Part model, mm, in its own coordinate system. A direction names the side the tool comes from. Give positions to 0.01 mm unless a question says otherwise; leave off trailing zeros. Loops run counter-clockwise (first coordinate to the right, second up) from the corner with the lowest first, then second, coordinate; pieces in that order, holes last. Notation, with made-up numbers: M -29.75,-3 L -5.75,-3 A15 ccw -5.75,26 Z; hole C -37,59.25 d2. An arc over 180 degrees is marked long. Answer in a Markdown table with one row per item.
from build123d import *

# Parameters (mm, degrees)
EXTRUDE_1_DEPTH     = 3.2
SKETCH_2_R          = 12.5
SKETCH_2_R_2        = 1.6
SKETCH_2_R_3        = 1.5
SKETCH_2_R_4        = 6.45
CUT_EXTRUDE_1_DEPTH = 3.2
FILLET_1_R          = 2
FILLET_2_R          = 1


# Read off the part's stored shape, not the designer's step: 凸台-拉伸1
with BuildPart() as part:
    # 凸台-拉伸1 outline → 凸台-拉伸1 (new body)
    with BuildSketch(Plane(origin=(0, 0, 0), x_dir=(1, 0, 0), z_dir=(0, 1, 0))):
        Polygon((-55, -0.171572875), (-66.828427125, -12), (-73, -12), (-73, -30), (73, -30), (73, -12), (66.828427125, -12), (55, -0.171572875), (55, 30), (-55, 30), align=None)
        Polygon((-64, -12), (-55, -3), (-55, -12), align=None, mode=Mode.SUBTRACT)
        Polygon((55, -12), (55, -3), (64, -12), align=None, mode=Mode.SUBTRACT)
    extrude(amount=EXTRUDE_1_DEPTH)

    # 草图2 → 切除-拉伸1 (cut)
    with BuildSketch(Plane(origin=(0, 3.2, 0), x_dir=(1, 0, 0), z_dir=(0, 1, 0))):
        with Locations(Location((0, -9.443650814, 0), (0, 0, 270))):
            Circle(SKETCH_2_R)
        with Locations(Location((15.556349186, -25, 0), (0, 0, 270))):
            Circle(SKETCH_2_R_2)
        with Locations(Location((15.556349186, 6.112698372, 0), (0, 0, 270))):
            Circle(SKETCH_2_R_2)
        with Locations(Location((-15.556349186, 6.112698372, 0), (0, 0, 270))):
            Circle(SKETCH_2_R_2)
        with Locations(Location((-15.556349186, -25, 0), (0, 0, 270))):
            Circle(SKETCH_2_R_2)
        with Locations(Location((-52.5, 20, 0), (0, 0, 270))):
            Circle(SKETCH_2_R_3)
        with Locations(Location((-52.5, -20, 0), (0, 0, 270))):
            Circle(SKETCH_2_R_3)
        with Locations(Location((52.5, -20, 0), (0, 0, 270))):
            Circle(SKETCH_2_R_3)
        with Locations(Location((52.5, 20, 0), (0, 0, 270))):
            Circle(SKETCH_2_R_3)
        with Locations(Location((-64, -21, 0), (0, 0, 270))):
            Circle(SKETCH_2_R_4)
        with Locations(Location((64, -21, 0), (0, 0, 270))):
            Circle(SKETCH_2_R_4)
        with Locations(Location((42, 20, 0), (0, 0, 270))):
            Circle(SKETCH_2_R_3)
        with Locations(Location((42, 12, 0), (0, 0, 270))):
            Circle(SKETCH_2_R_3)
        with Locations(Location((-42, 12, 0), (0, 0, 270))):
            Circle(SKETCH_2_R_3)
        with Locations(Location((-42, 20, 0), (0, 0, 270))):
            Circle(SKETCH_2_R_3)
        with Locations(Location((42, -11, 0), (0, 0, 270))):
            Circle(SKETCH_2_R_3)
        with Locations(Location((-42, -11, 0), (0, 0, 270))):
            Circle(SKETCH_2_R_3)
        with Locations(Location((-28.065, 27, 0), (0, 0, 270))):
            Circle(SKETCH_2_R_3)
        with Locations(Location((28.065, 27, 0), (0, 0, 270))):
            Circle(SKETCH_2_R_3)
        with Locations(Location((-28.065, -16.18, 0), (0, 0, 270))):
            Circle(SKETCH_2_R_3)
        with Locations(Location((28.065, -16.18, 0), (0, 0, 270))):
            Circle(SKETCH_2_R_3)
        with Locations(Location((-28.769, -27.5, 0), (0, 0, 270))):
            Circle(SKETCH_2_R_3)
        with Locations(Location((28.769, -27.5, 0), (0, 0, 270))):
            Circle(SKETCH_2_R_3)
        with Locations(Location((-44.769, -20, 0), (0, 0, 270))):
            Circle(SKETCH_2_R_3)
        with Locations(Location((44.769, -20, 0), (0, 0, 270))):
            Circle(SKETCH_2_R_3)
    extrude(amount=-CUT_EXTRUDE_1_DEPTH, mode=Mode.SUBTRACT)

    # 圆角1
    fillet_1_edges = [part.edges().sort_by_distance(p)[0] for p in [
        (-66.828427125, 1.6, 12),
        (-55, 1.6, 0.171572875),
        (-55, 1.6, -30),
        (55, 1.6, -30),
        (55, 1.6, 0.171572875),
        (66.828427125, 1.6, 12),
        (73, 1.6, 12),
        (73, 1.6, 30),
        (-73, 1.6, 30),
        (-73, 1.6, 12),
    ]]
    fillet(fillet_1_edges, radius=FILLET_1_R)

    # 圆角2
    fillet_2_edges = [part.edges().sort_by_distance(p)[0] for p in [
        (-64, 1.6, 12),
        (-55, 1.6, 12),
        (-55, 1.6, 3),
        (55, 1.6, 3),
        (55, 1.6, 12),
        (64, 1.6, 12),
    ]]
    fillet(fillet_2_edges, radius=FILLET_2_R)


solid = part.part
(1) Pin check, flat tips, straight feed: pin 1 Ø7.5 at (x, z) = (-64, 21) entering from -Y; pin 2 Ø1.6 at (y, z) = (2, -15.5) entering from +X. Stop position of each tip, or through.
Recorded:
| item | result |
|---|---|
| pin 1 | passes through |
| pin 2 | stops at x = 55 |
(2) Saw through at C-C (x = -64). Write the cut outline in (y, z), plus the area to 3 significant figures.
Recorded:
| item | result |
|---|---|
| outline | M 0,9.17 L 3.2,9.17 L 3.2,14.55 L 0,14.55 Z; M 0,27.45 L 3.2,27.45 L 3.2,30 L 0,30 Z |
| area | 25.4 mm^2 |
(3) Pull direction Z, two halves, no side cores. Call faces 3 (the face through (55, 2, 8)), 4 (the face through (-1, 0, -7)), 5 (the face through (-1, 2, 30)): +Z half, -Z half, draft (parallel to the pull), parting line (faces both ways), or undercut.
Recorded:
| item | result |
|---|---|
| face 3 | undercut |
| face 4 | draft |
| face 5 | +Z half |
(4) Which spindle directions (+Z, -Z, +X, -X, +Y, -Y) get a long thin tool onto all of the face, cutting with end or side? Do faces 1 (the face through (73, 2, 21)), 2 (the face through (59, 2, 7)). Say none if no direction does.
Recorded:
| item | result |
|---|---|
| face 1 | +Z, -Z, +X, +Y, -Y |
| face 2 | +Y, -Y |
(5) Saw through at A-A (z = -12). Write the cut outline in (x, y), plus the area to 3 significant figures.
Recorded:
| item | result |
|---|---|
| outline | M -55,0 L -43.5,0 L -43.5,3.2 L -55,3.2 Z; M -40.5,0 L 40.5,0 L 40.5,3.2 L -40.5,3.2 Z; M 43.5,0 L 55,0 L 55,3.2 L 43.5,3.2 Z |
| area | 333 mm^2 |
(6) Drill centre lines: line 1 along X through (y, z) = (1, -20); line 2 along X through (y, z) = (1.2, -27) (3 decimals); line 3 along X through (y, z) = (1.85, 27.5). Where is each one in solid material? Low to high.
Recorded:
| item | result |
|---|---|
| line 1 | x = -55 to -54, -51 to -43.5, -40.5 to 40.5, 43.5 to 51, 54 to 55 |
| line 2 | x = -55 to -29.565, -26.565 to 26.565, 29.565 to 55 |
| line 3 | x = -73 to -30.27, -27.27 to 27.27, 30.27 to 73 |
(7) Saw through at B-B (x = 42). Write the cut outline in (y, z), plus the area to 3 significant figures.
Recorded:
| item | result |
|---|---|
| outline | M 0,-30 L 3.2,-30 L 3.2,-21.5 L 0,-21.5 Z; M 0,-18.5 L 3.2,-18.5 L 3.2,-13.5 L 0,-13.5 Z; M 0,-10.5 L 3.2,-10.5 L 3.2,9.5 L 0,9.5 Z; M 0,12.5 L 3.2,12.5 L 3.2,30 L 0,30 Z |
| area | 163 mm^2 |
(8) Saw through at D-D (z = 20). Give the number of separate pieces and of enclosed holes in the cut face, plus the area to 3 significant figures.
Recorded:
| item | result |
|---|---|
| separate pieces | 8 |
| enclosed holes | 0 |
| area | 304 mm^2 |
